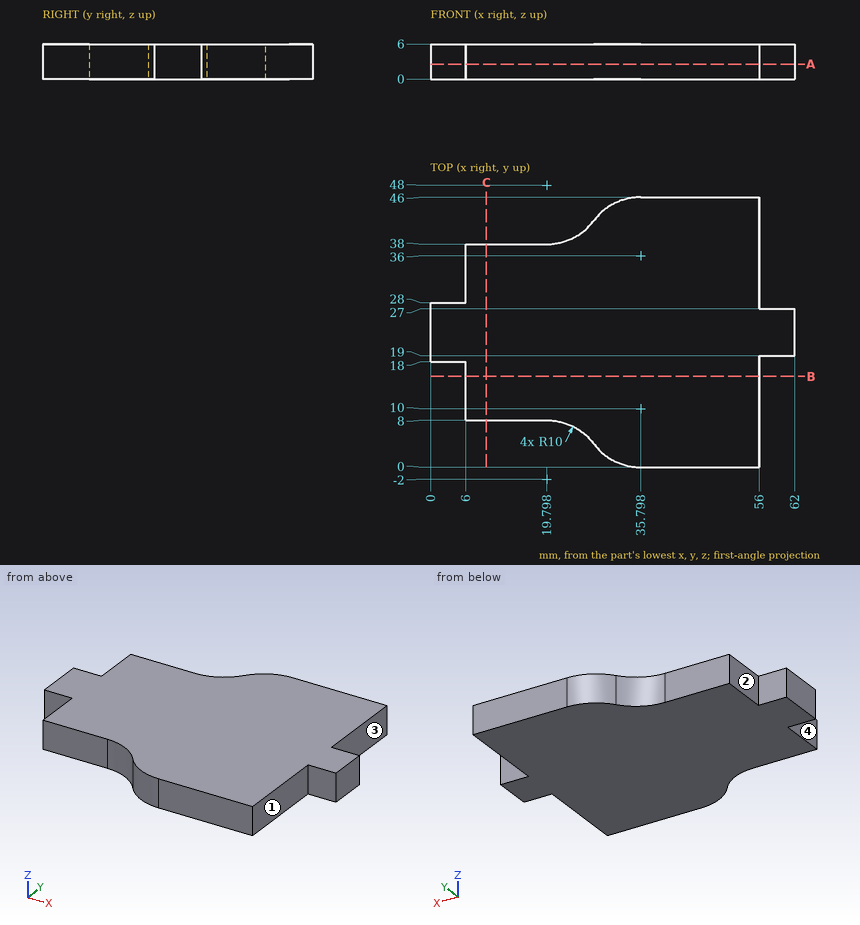
Print and shaded views of the part. All mm, measured from the part's lowest x, y and z. A direction names the side the tool comes from. Round coordinates to 2 decimals unless told otherwise and drop trailing zeros. Write each loop counter-clockwise with the first axis right and the second up, starting at its lowest first coordinate (ties: lowest second). Pieces come first, ordered by that corner, then holes. Notation, with made-up numbers: (-34, 37) -> (16, 37) arc R13 cw to (16, 41) -> close; hole circle Ø3 at (-39, 29). An arc over 180 degrees is marked (long way). Return JSON: item names as keys, results as strings. Group by question number.
Q1. Saw through at B-B on y = 15.5. Write the cut outline in (x, z).
Q2. Pin check, flat tips, straight feed: pin 1 (3 mm diameter, centred on y = 9, z = 4.5, fed in from +X); pin 2 (1 mm diameter, centred on x = 25, z = 1, fed in from +Y) (3 decimals); pin 3 (1.8 mm diameter, centred on x = 4, z = 2, fed in from +Y); pin 4 (3 mm diameter, centred on x = 13, y = 41, fed in from +Z). Stop position of each tip, or through.
Q3. Probe L1, parallel to Y at x = 57.5, z = 3.3; L2, parallel to X at y = 14, z = 5.6; L3, parallel to Y at x = 8.5, z = 1.05. List the from-to ranges inside material, lowest first. Write a range as [from, to].
Q4. Saw through at C-C on x = 9.5. Write the cut outline in (y, z).
Q5. Which spindle directions (+Z, -Z, +X, -X, +Y, -Y) get a long thin tool onto all of the face, cutting with end or side? Do the marked faces 1, 2, 3 and 4. Say none if no direction does.
Q6. Saw through at A-A on z = 2.55. Write the cut outline in (x, y), plus the area to 3 significant figures.
Answer:
{
 "1": {"outline": "(6, 0) -> (56, 0) -> (56, 6) -> (6, 6) -> close"},
 "2": {"pin 1": "x = 56", "pin 2": "y = 39.785", "pin 3": "y = 28", "pin 4": "through"},
 "3": {"L1": "[19, 27]", "L2": "[6, 56]", "L3": "[8, 38]"},
 "4": {"outline": "(8, 0) -> (38, 0) -> (38, 6) -> (8, 6) -> close"},
 "5": {"face 1": "+Z, -Z, +X, -Y", "face 2": "+Z, -Z, -X, +Y", "face 3": "+Z, -Z, +X, +Y", "face 4": "+Z, -Z, -X, -Y"},
 "6": {"outline": "(0, 18) -> (6, 18) -> (6, 8) -> (19.8, 8) arc R10 cw to (27.8, 4) arc R10 ccw to (35.8, 0) -> (56, 0) -> (56, 19) -> (62, 19) -> (62, 27) -> (56, 27) -> (56, 46) -> (35.8, 46) arc R10 ccw to (27.8, 42) arc R10 cw to (19.8, 38) -> (6, 38) -> (6, 28) -> (0, 28) -> close", "area": "2,060 mm2"}
}
